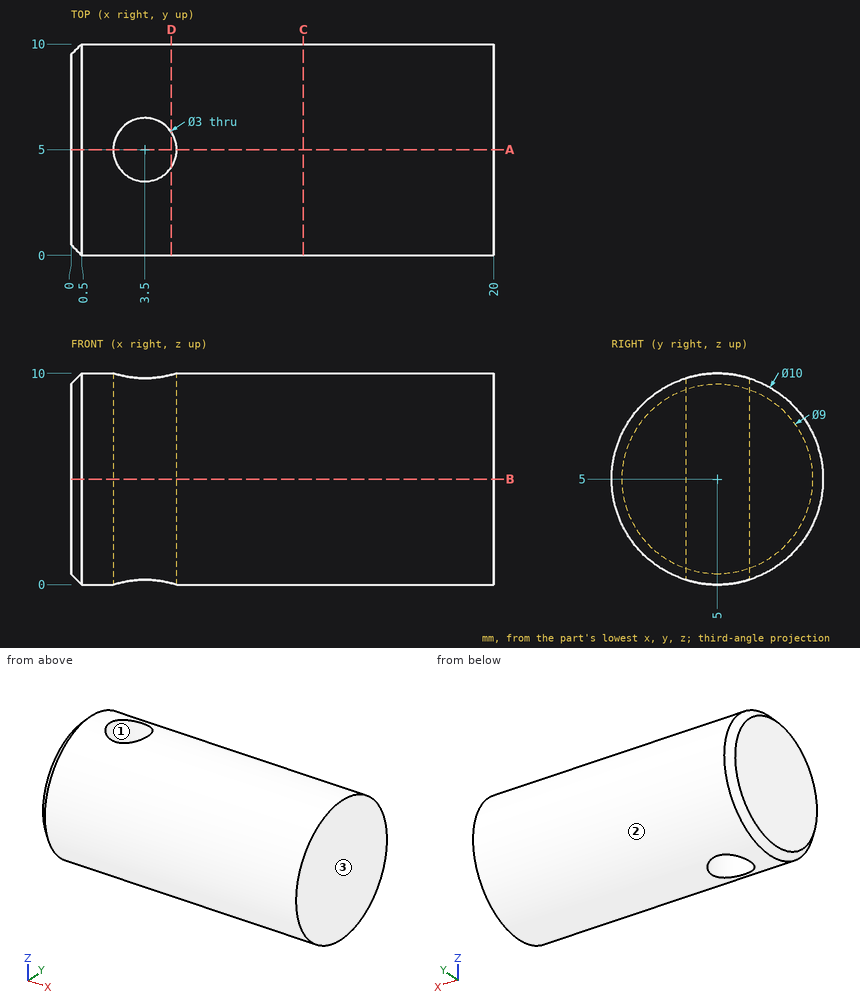
Check sheet for the drawn part. Datum: minimum x, y, z corner. Units: mm. Give positions to 0.01 mm unless a question says otherwise; leave off trailing zeros. Write each loop counter-clockwise with the first axis right and the second up, starting at its lowest first coordinate (ties: lowest second). Pieces come first, ordered by that corner, then holes. Notation, with made-up numbers: M 33.5,52 L 78.5,52 A35 ccw 78.5,85 Z; hole C -38,23.5 d1. An arc over 180 degrees is marked long. Write item = value, one per line.
(1) Sectioned sample at A-A (y = 5). Record the cut outline in (x, z).
Found:
outline = M 0,0.5 L 0.5,0 L 2,0 L 2,10 L 0.5,10 L 0,9.5 Z; M 5,0 L 20,0 L 20,10 L 5,10 Z
(2) Sectioned sample at C-C (x = 11). Record the cut outline in (y, z).
Found:
outline = C 5,5 d10
(3) Material ranges on line 1 (X direction, y = 4.5, z = 8); line 2 (Y direction, x = 2.5, z = 4); line 3 (Y direction, x = 3.5, z = 4.75), recorded low to high.
Found:
line_1 = 0 to 2.09, 4.91 to 20
line_2 = 0.1 to 3.88, 6.12 to 9.9
line_3 = 0.01 to 3.5, 6.5 to 9.99
(4) Sectioned sample at D-D (x = 4.75). Record the cut outline in (y, z), then the cut area to 3 significant figures.
Found:
outline = M 4.17,0.07 L 4.17,9.93 A5 ccw Z; M 5.83,0.07 A5 ccw 5.83,9.93 Z
area = 62.0 mm2
(5) Go/stop test with flat-tipped pins: pin 1 Ø1.5 at (x, y) = (7.5, 4) entering from +Z; pin 2 Ø2 at (x, y) = (14, 9) entering from +Z; pin 3 Ø5 at (x, z) = (15.5, 1.5) entering from +Y. Record where each tip stops, or that it passes through.
Found:
pin_1 = 9.99
pin_2 = 9
pin_3 = 9.9
(6) Draft check along Y on the marked faces 1, 2 and 3. Enter one of: released by +Y, released by -Y, zero draft, split by the parting line, or undercut.
Found:
face_1 = undercut
face_2 = split by the parting line
face_3 = zero draft
(7) Sectioned sample at B-B (z = 5). Record the cut outline in (x, y), then the cut area to 3 significant figures.
Found:
outline = M 0,0.5 L 0.5,0 L 20,0 L 20,10 L 0.5,10 L 0,9.5 Z; hole C 3.5,5 d3
area = 193 mm2
